Geometry: final body of the model. Coordinates: model frame, mm. A direction names the side the tool comes from. Give positions to 0.01 mm unless a question says otherwise; leave off trailing zeros. Write each loop counter-clockwise with the first axis right and the second up, starting at its lowest first coordinate (ties: lowest second). Pieces come first, ordered by that corner, then holes.
Q1. Cut plane C-C on y = 202. Return the cut outline in (x, z).
Q2. Pin query (flat end, axial travel): pin 1 (9.5 mm diameter, centred on x = 115, z = -11.5, fed in from +Y); pin 2 (1.5 mm diameter, centred on x = 172, z = -12.5, fed in from -Y); pin 3 (8 mm diameter, centred on x = 108.5, y = 80.5, fed in from +Z); pin 4 (5.5 mm diameter, centred on y = -10.5, z = -6.5, fed in from +X). Return the tip coordinate at first contact, or that it passes through.
Q3. Cut plane A-A on z = -3. Count the separate pieces of the cut face and the enclosed holes in it, plus the area to 3 significant figures.
Q4. Line query: L1, parallel to X at y = 79.5, z = -7.75; L2, parallel to X at y = 225, z = -6; L3, parallel to Y at x = 215, z = -15.75. Output: solid intervals per line, ascending.
Q5. Cut plane B-B on x = 189.5. Return the cut outline in (y, z), plus the area to 3 significant figures.
Q6. Reachability of faces 4 (the face through (13, 0, -9)), 5 (the face through (25.4, 232, -9)), 6 (the face through (361.95, 143, -9)), 7 (the face through (361.95, 19, -9)) from +Z, -Z, +X, -X, +Y, -Y: full face, straight path, thin tool, end or side. Return the list, or none.
Q7. Draft query along X for faces 1 (the face through (146.05, -9, -9)), 2 (the face through (44.45, -9, -9)), 3 (the face through (252, 222.25, -9)). Return one class per face: pulls with the +X half, pulls with the -X half, needs draft (parallel to the pull), parting line crosses it, or undercut.
```python
from build123d import *

# Parameters (mm, degrees)
SKETCH1_W               = 361.95
SKETCH1_H               = 222.25
BOSS_EXTRUDE1_DEPTH     = 19.05
SKETCH3_W               = 19.05
SKETCH3_H               = 19.05
BOSS_EXTRUDE4_DEPTH     = 19.05
SKETCH5_W               = 19.05
SKETCH5_H               = 19.05
BOSS_EXTRUDE5_DEPTH     = 19.05
CUT_EXTRUDE2_DEPTH      = 452.386300745
CUT_EXTRUDE2_DEPTH_BACK = 452.386300745


with BuildPart() as part:
    # Sketch1 → Boss-Extrude1 (new body)
    with BuildSketch(Plane.XY):
        with Locations((180.975, 111.125)):
            Rectangle(SKETCH1_W, SKETCH1_H)
    extrude(amount=-BOSS_EXTRUDE1_DEPTH)

    # Sketch3 → Boss-Extrude4 (add)
    with BuildSketch(Plane.XY):
        with Locations((34.925, 231.775)):
            Rectangle(SKETCH3_W, SKETCH3_H)
        with Locations((85.725, 231.775)):
            Rectangle(SKETCH3_W, SKETCH3_H)
        with Locations((136.525, 231.775)):
            Rectangle(SKETCH3_W, SKETCH3_H)
    boss_extrude4 = extrude(amount=-BOSS_EXTRUDE4_DEPTH)

    # Mirror1: Boss-Extrude4 across plane
    add(boss_extrude4.mirror(Plane.ZX.offset(111.125)))

    # Sketch5 → Boss-Extrude5 (add)
    with BuildSketch(Plane.XY):
        with Locations((371.475, 174.625)):
            Rectangle(SKETCH5_W, SKETCH5_H)
        with Locations((371.475, 47.625)):
            Rectangle(SKETCH5_W, SKETCH5_H)
        with Locations((371.475, 111.125)):
            Rectangle(SKETCH5_W, SKETCH5_H)
    extrude(amount=-BOSS_EXTRUDE5_DEPTH)

    # Sketch6 → Cut-Extrude2 (cut, two sides: drawn at the far end of the back side and taken through both)
    with BuildSketch(Plane.XY.offset(-CUT_EXTRUDE2_DEPTH_BACK)):
        with BuildLine():
            Line((85.725, 88.9), (92.075, 88.9))
            ThreePointArc((92.075, 88.9), (97.49506403, 91.14506403), (95.25, 85.725))
            Line((95.25, 85.725), (95.25, 79.375))
            ThreePointArc((95.25, 79.375), (97.49506403, 73.95493597), (92.075, 76.2))
            Line((92.075, 76.2), (85.725, 76.2))
            ThreePointArc((85.725, 76.2), (80.30493597, 73.95493597), (82.55, 79.375))
            Line((82.55, 79.375), (82.55, 85.725))
            ThreePointArc((82.55, 85.725), (80.30493597, 91.14506403), (85.725, 88.9))
        make_face()
        with BuildLine():
            Line((149.225, 76.2), (155.575, 76.2))
            ThreePointArc((155.575, 76.2), (160.99506403, 73.95493597), (158.75, 79.375))
            Line((158.75, 79.375), (158.75, 85.725))
            ThreePointArc((158.75, 85.725), (160.99506403, 91.14506403), (155.575, 88.9))
            Line((155.575, 88.9), (149.225, 88.9))
            ThreePointArc((149.225, 88.9), (143.80493597, 91.14506403), (146.05, 85.725))
            Line((146.05, 85.725), (146.05, 79.375))
            ThreePointArc((146.05, 79.375), (143.80493597, 73.95493597), (149.225, 76.2))
        make_face()
        with BuildLine():
            Line((212.725, 76.2), (219.075, 76.2))
            ThreePointArc((219.075, 76.2), (224.49506403, 73.95493597), (222.25, 79.375))
            Line((222.25, 79.375), (222.25, 85.725))
            ThreePointArc((222.25, 85.725), (224.49506403, 91.14506403), (219.075, 88.9))
            Line((219.075, 88.9), (212.725, 88.9))
            ThreePointArc((212.725, 88.9), (207.30493597, 91.14506403), (209.55, 85.725))
            Line((209.55, 85.725), (209.55, 79.375))
            ThreePointArc((209.55, 79.375), (207.30493597, 73.95493597), (212.725, 76.2))
        make_face()
        with BuildLine():
            Line((276.225, 76.2), (282.575, 76.2))
            ThreePointArc((282.575, 76.2), (287.99506403, 73.95493597), (285.75, 79.375))
            Line((285.75, 79.375), (285.75, 85.725))
            ThreePointArc((285.75, 85.725), (287.99506403, 91.14506403), (282.575, 88.9))
            Line((282.575, 88.9), (276.225, 88.9))
            ThreePointArc((276.225, 88.9), (270.80493597, 91.14506403), (273.05, 85.725))
            Line((273.05, 85.725), (273.05, 79.375))
            ThreePointArc((273.05, 79.375), (270.80493597, 73.95493597), (276.225, 76.2))
        make_face()
        with BuildLine():
            Line((149.225, 152.4), (155.575, 152.4))
            ThreePointArc((155.575, 152.4), (160.99506403, 150.15493597), (158.75, 155.575))
            Line((158.75, 155.575), (158.75, 161.925))
            ThreePointArc((158.75, 161.925), (160.99506403, 167.34506403), (155.575, 165.1))
            Line((155.575, 165.1), (149.225, 165.1))
            ThreePointArc((149.225, 165.1), (143.80493597, 167.34506403), (146.05, 161.925))
            Line((146.05, 161.925), (146.05, 155.575))
            ThreePointArc((146.05, 155.575), (143.80493597, 150.15493597), (149.225, 152.4))
        make_face()
        with BuildLine():
            Line((212.725, 152.4), (219.075, 152.4))
            ThreePointArc((219.075, 152.4), (224.49506403, 150.15493597), (222.25, 155.575))
            Line((222.25, 155.575), (222.25, 161.925))
            ThreePointArc((222.25, 161.925), (224.49506403, 167.34506403), (219.075, 165.1))
            Line((219.075, 165.1), (212.725, 165.1))
            ThreePointArc((212.725, 165.1), (207.30493597, 167.34506403), (209.55, 161.925))
            Line((209.55, 161.925), (209.55, 155.575))
            ThreePointArc((209.55, 155.575), (207.30493597, 150.15493597), (212.725, 152.4))
        make_face()
        with BuildLine():
            Line((276.225, 152.4), (282.575, 152.4))
            ThreePointArc((282.575, 152.4), (287.99506403, 150.15493597), (285.75, 155.575))
            Line((285.75, 155.575), (285.75, 161.925))
            ThreePointArc((285.75, 161.925), (287.99506403, 167.34506403), (282.575, 165.1))
            Line((282.575, 165.1), (276.225, 165.1))
            ThreePointArc((276.225, 165.1), (270.80493597, 167.34506403), (273.05, 161.925))
            Line((273.05, 161.925), (273.05, 155.575))
            ThreePointArc((273.05, 155.575), (270.80493597, 150.15493597), (276.225, 152.4))
        make_face()
        with BuildLine():
            Line((85.725, 152.4), (92.075, 152.4))
            ThreePointArc((92.075, 152.4), (97.49506403, 150.15493597), (95.25, 155.575))
            Line((95.25, 155.575), (95.25, 161.925))
            ThreePointArc((95.25, 161.925), (97.49506403, 167.34506403), (92.075, 165.1))
            Line((92.075, 165.1), (85.725, 165.1))
            ThreePointArc((85.725, 165.1), (80.30493597, 167.34506403), (82.55, 161.925))
            Line((82.55, 161.925), (82.55, 155.575))
            ThreePointArc((82.55, 155.575), (80.30493597, 150.15493597), (85.725, 152.4))
        make_face()
    extrude(amount=CUT_EXTRUDE2_DEPTH + CUT_EXTRUDE2_DEPTH_BACK, mode=Mode.SUBTRACT)


solid = part.part
```
Data:
1. outline: (0, -19.05) - (361.95, -19.05) - (361.95, 0) - (0, 0) - close
2. pin 1: stops at y = 222.25
2. pin 2: stops at y = 0
2. pin 3: stops at z = 0
2. pin 4: stops at x = 146.05
3. separate pieces: 1
3. enclosed holes: 8
3. area: 81,700 mm2
4. L1: x = 0 to 82.55, 95.25 to 146.05, 158.75 to 209.55, 222.25 to 273.05, 285.75 to 361.95
4. L2: x = 25.4 to 44.45, 76.2 to 95.25, 127 to 146.05
4. L3: y = 0 to 76.2, 88.9 to 152.4, 165.1 to 222.25
5. outline: (0, -19.05) - (222.25, -19.05) - (222.25, 0) - (0, 0) - close
5. area: 4,230 mm2
6. face 4: +Z, -Z, -X, -Y
6. face 5: +Z, -Z, -X, +Y
6. face 6: +Z, -Z, +X
6. face 7: +Z, -Z, +X, -Y
7. face 1: pulls with the +X half
7. face 2: undercut
7. face 3: needs draft
